The listing builds one solid part. Answer for the finished solid, in the listing's coordinates (mm). A direction names the side the tool comes from. Round coordinates to 2 decimals unless told otherwise and drop trailing zeros. Write each loop counter-clockwise with the first axis right and the second up, starting at its lowest first coordinate (ties: lowest second). Pieces come first, ordered by that corner, then holes. Notation, with made-up numbers: (75, 81) - (108, 81) arc R14 ccw to (108, 94) - close; hole circle Ø11 at (24.5, 39). An arc over 180 degrees is marked (long way). Answer in a Markdown table with one row per item.
Autodesk Inventor part; units mm, degrees
ref_plane "YZ Plane" through (0, 0, 0) normal (1, 0, 0) x (0, 1, 0)
ref_plane "XZ Plane" through (0, 0, 0) normal (0, 1, 0) x (-1, 0, 0)
ref_plane "XY Plane" through (0, 0, 0) normal (0, 0, 1) x (1, 0, 0)
sketch "Sketch1" plane through (0, 0, 0) normal (0, 0, 1) x (1, 0, 0)
  line L0 (-100, -125) -> (100, -125)
  line L1 (100, -125) -> (100, 125)
  line L2 (100, 125) -> (-100, 125)
  line L3 (-100, 125) -> (-100, -125)
  line L4 (-100, -125) -> (100, 125) construction
  line L5 (100, -125) -> (-100, 125) construction
  point P0 (0, 0)
  dimension "Height" = 250
  dimension "Width" = 200
extrude "Extrusion1" add sketch "Sketch1" along normal blind 19.05
sketch "Sketch2" plane through (0, 0, 19.05) normal (0, 0, 1) x (1, 0, 0)
  line L0 (-30, 90) -> (30, 90) construction
  line L1 (-30, 80) -> (30, 80)
  line L2 (30, 100) -> (-30, 100)
  arc A0 (-30, 100) -> (-30, 80) centre (-30, 90) ccw
  arc A1 (30, 80) -> (30, 100) centre (30, 90) ccw
  line L3 (100, 125) -> (-100, 125)
  point P0 (0, 0)
  point P1 (0, 90)
  dimension "d4" = 30
  dimension "d5" = 20
  dimension "d6" = 25
extrude "Extrusion2" cut sketch "Sketch2" against normal up to surface (19.05 mm away)
equation "\"d7\" = thickness"
properties part number "Creat Side" material "Wood (Cherry)"
(1) For a pull along X with two mould halves and no side action, classify faces 3 (the flat face through (-100, 2, 9)), 4 (the cylindrical face through (-40, 90, 10)), 5 (the flat face through (1, 125, 9)), 6 (the flat face through (100, -2, 9)) as pulls with the +X half, pulls with the -X half, needs draft (parallel to the pull), parting line crosses it, or undercut.
Checked values:
| item | result |
|---|---|
| face 3 | pulls with the -X half |
| face 4 | undercut |
| face 5 | needs draft |
| face 6 | pulls with the +X half |
(2) Section A-A (x = 1.5) is taken. Give the vertices of the cut face in (y, z), and give its area (3 significant figures).
Checked values:
| item | result |
|---|---|
| outline | (-125, 0) - (80, 0) - (80, 19.05) - (-125, 19.05) - close; (100, 0) - (125, 0) - (125, 19.05) - (100, 19.05) - close |
| area | 4,380 mm2 |
(3) Section C-C (z = 4.75) is taken. Give the vertices of the cut face in (x, y).
Checked values:
| item | result |
|---|---|
| outline | (-100, -125) - (100, -125) - (100, 125) - (-100, 125) - close; hole (-30, 80) - (30, 80) arc R10 ccw to (30, 100) - (-30, 100) arc R10 ccw to start |
(4) Flat-ended cylindrical pins translate along their axes: pin 1 (10 mm diameter, centred on x = -4.5, y = 23, fed in from -Z); pin 2 (5 mm diameter, centred on x = 18.5, y = 84, fed in from +Z). Find the tip coordinate at first contact, or state that the pin passes through.
Checked values:
| item | result |
|---|---|
| pin 1 | stops at z = 0 |
| pin 2 | passes through |
(5) Section B-B (y = 90) is taken. Give the vertices of the cut face in (x, z), and give its area (3 significant figures).
Checked values:
| item | result |
|---|---|
| outline | (-100, 0) - (-40, 0) - (-40, 19.05) - (-100, 19.05) - close; (40, 0) - (100, 0) - (100, 19.05) - (40, 19.05) - close |
| area | 2,290 mm2 |
(6) For faces 1 (the flat face through (-1, 2, 0)), 2 (the flat face through (0, 80, 10)), determine the directions among +Z, -Z, +X, -X, +Y, -Y from which every point of the face is accessible in a straight line to the end or side of a thin tool.
Checked values:
| item | result |
|---|---|
| face 1 | -Z, +X, -X, +Y, -Y |
| face 2 | +Z, -Z |
(7) Find the intervals of material crossed by line 1 (Y direction, x = -20.5, z = 15); line 2 (Y direction, x = -31.5, z = 11.5), in increasing order.
Checked values:
| item | result |
|---|---|
| line 1 | y = -125 to 80, 100 to 125 |
| line 2 | y = -125 to 80.11, 99.89 to 125 |
